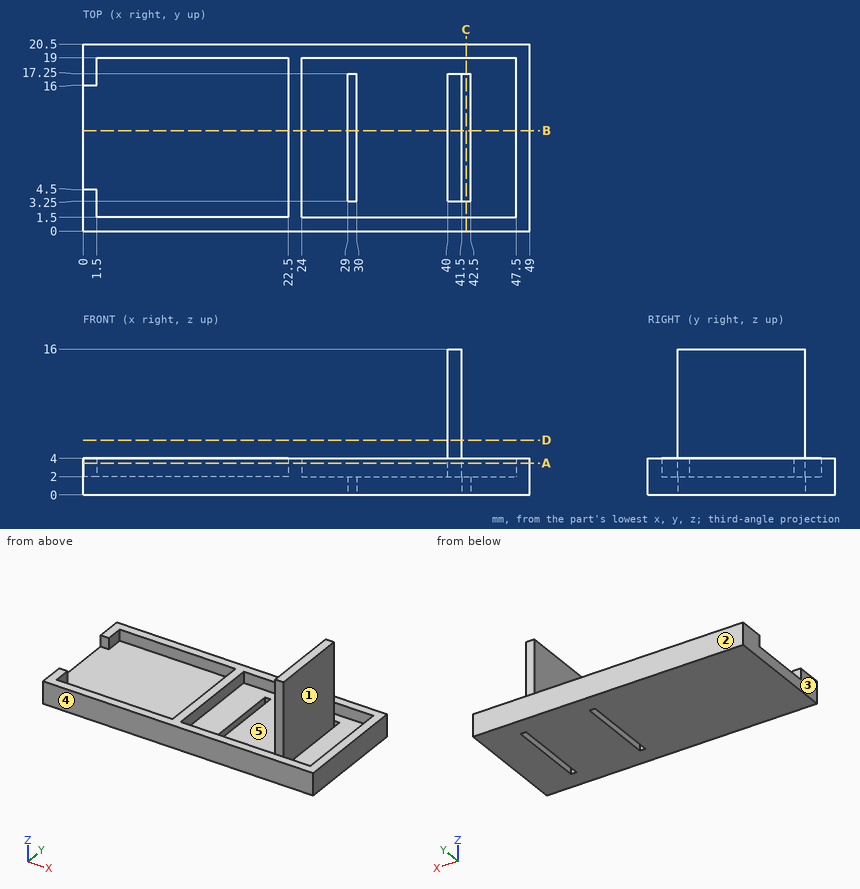
The drawing under review shows one solid part. Ordinate dimensions are in mm from its lowest x, y, z. A direction names the side the tool comes from. Coordinates: 2 decimals unless noted, no trailing zeros. Write each loop counter-clockwise with the first axis right and the second up, starting at its lowest first coordinate (ties: lowest second). Pieces come first, ordered by that corner, then holes. Notation, with made-up numbers: (1, 46.25) - (17, 46.25) arc R20 cw to (17, 72.25) - close; hole circle Ø6 at (86, -30). An arc over 180 degrees is marked (long way). Answer in a Markdown table with one row per item. Add a question column.
Q1. Draft analysis for pull direction Y (two halves, no side actions). For the marked faces 3, 4 and 5, state which applies: +Y half, -Y half, draft (parallel to the pull), parting line (faces both ways), or undercut.
Q2. For probe 1 along X at (y, z) = (10.5, 3); probe 2 along X at (y, z) = (10.75, 11.5); probe 3 along Z at (x, y) = (20, 13.25), list the stretches that pass through material, from the lowest coordinate up.
Q3. We need section D-D, the plane z = 6. State the section outline as (x, y) points.
Q4. We need section B-B, the plane y = 11. State the section outline as (x, z) points, and give its area (3 significant figures).
Q5. Tool access review of the marked faces 1 and 2: name each direction out of +Z, -Z, +X, -X, +Y, -Y from which nothing blocks a thin tool from reaching the whole face with its end or side.
Q6. We need section A-A, the plane z = 3.5. State the section outline as (x, y) points, and give its area (4 significant figures).
Q7. For P1, Ø4, axis at y = 13, z = 8, coming from the -X side; P2, Ø4, axis at x = 6, y = 8.5, coming from the +Z side; P3, Ø1, axis at y = 6.5, z = 3.5, coming from the -X side, all flat-tipped, find the tip position at first contact; note any pin that passes through.
Q8. We need section C-C, the plane x = 42. State the section outline as (y, z) points, and give its area (3 significant figures).
Answer list:
| question | item | result |
|---|---|---|
| 1 | face 3 | draft |
| 1 | face 4 | -Y half |
| 1 | face 5 | undercut |
| 2 | probe 1 | x = 22.5 to 24, 40 to 41.5, 47.5 to 49 |
| 2 | probe 2 | x = 40 to 41.5 |
| 2 | probe 3 | z = 0 to 2 |
| 3 | outline | (40, 3.25) - (41.5, 3.25) - (41.5, 17.25) - (40, 17.25) - close |
| 4 | outline | (0, 0) - (29, 0) - (29, 2) - (24, 2) - (24, 4) - (22.5, 4) - (22.5, 2) - (0, 2) - close; (30, 0) - (41.5, 0) - (41.5, 16) - (40, 16) - (40, 2) - (30, 2) - close; (42.5, 0) - (49, 0) - (49, 4) - (47.5, 4) - (47.5, 2) - (42.5, 2) - close |
| 4 | area | 121 mm2 |
| 5 | face 1 | +Z, -Z |
| 5 | face 2 | +Z, -Z, +X, -X, +Y |
| 6 | outline | (0, 0) - (49, 0) - (49, 20.5) - (0, 20.5) - (0, 16) - (1.5, 16) - (1.5, 19) - (22.5, 19) - (22.5, 1.5) - (1.5, 1.5) - (1.5, 4.5) - (0, 4.5) - close; (40, 3.25) - (41.5, 3.25) - (41.5, 17.25) - (40, 17.25) - close; hole (24, 1.5) - (47.5, 1.5) - (47.5, 19) - (24, 19) - close |
| 6 | area | 229.5 mm2 |
| 7 | P1 | stops at x = 40 |
| 7 | P2 | stops at z = 2 |
| 7 | P3 | stops at x = 22.5 |
| 8 | outline | (0, 0) - (3.25, 0) - (3.25, 2) - (1.5, 2) - (1.5, 4) - (0, 4) - close; (17.25, 0) - (20.5, 0) - (20.5, 4) - (19, 4) - (19, 2) - (17.25, 2) - close |
| 8 | area | 19.0 mm2 |
